from build123d import *

# Parameters (mm, degrees)
F1_DEPTH = 10
F2_DEPTH = 25
F3_R     = 7
F4_DEPTH = 60
F5_R     = 5


with BuildPart() as f1:
    # F0 (on Top) → F1 (new body)
    with BuildSketch(Plane.XY):
        Polygon((-115.381198, -8), (-4.618802, -8), (-9.237604, 0), (-4.618802, 8), (-115.381198, 8), align=None)
    extrude(amount=-F1_DEPTH)

    # F0 (on Top) → F2 (join)
    with BuildSketch(Plane.XY):
        Polygon((4.618802, -8), (9.237604, 0), (4.618802, 8), (-4.618802, 8), (-9.237604, 0), (-4.618802, -8), align=None)
        Polygon((2.453739, 4.25), (4.907477, 0), (2.453739, -4.25), (-2.453739, -4.25), (-4.907477, 0), (-2.453739, 4.25), align=None, mode=Mode.SUBTRACT)
    extrude(amount=-F2_DEPTH)

    # F3 (on face) → F4 (join)
    with BuildSketch(Plane(origin=(0, 0, -10), x_dir=(1, 0, 0), z_dir=(0, 0, -1))):
        with Locations((-107.381198, 0)):
            Circle(F3_R)
    extrude(amount=-F4_DEPTH)

    # F5
    f5_edges = [f1.edges().sort_by_distance(p)[0] for p in [
        (-114.381198, 0, 50),
    ]]
    fillet(f5_edges, radius=F5_R)


solid = f1.part
Work out the finished part from the listing and answer in its coordinate system (mm). A direction names the side the tool comes from. Give positions to 0.01 mm unless a question says otherwise; leave off trailing zeros. Loops run counter-clockwise (first coordinate to the right, second up) from the corner with the lowest first, then second, coordinate; pieces in that order, holes last. Notation, with made-up numbers: (-5.5, 58) -> (30.5, 58) arc R32 ccw to (30.5, 93) -> close; hole circle Ø5 at (73, 48.25). An arc over 180 degrees is marked (long way). Use a Markdown table: item, result. Add a question column.
1. Find the intervals of material crossed by probe 1 along Z at (x, y) = (-3, -5.5); probe 2 along Z at (x, y) = (-81, 7); probe 3 along X at (y, z) = (-0.5, -11), in increasing order.
2. For faces 4 (the flat face through (-6.896, 4.056, -17.395)), 5 (the flat face through (-6.961, -3.944, -17.395)), 6 (the cylindrical face through (-114.374, -0.308, 22.185)), 7 (the flat face through (-3.698, 2.095, -12.325)), 8 (the flat face through (-55, 8, -7)), determine the directions among +Z, -Z, +X, -X, +Y, -Y from which every point of the face is accessible in a straight line to the end or side of a thin tool.
3. Determine the mould class of faces 1 (the flat face through (-3.663, -2.155, -12.325)), 2 (the flat face through (4, 2, -25)), 3 (the flat face through (-115.381, 0, -5)) for opening direction X: released by +X, released by -X, zero draft, split by the parting line, or undercut.
4. Flat-ended cylindrical pins translate along their axes: pin 1 Ø6 at (y, z) = (0.5, 5) entering from -X; pin 2 Ø8 at (y, z) = (-6, 31) entering from +X; pin 3 Ø4 at (x, y) = (-53, 5) entering from -Z; pin 4 Ø6 at (x, y) = (-9, 4) entering from -Z. Find the tip coordinate at first contact, or state that the pin passes through.
5. Section A-A on x = -86.5 is taken. Determine the outline of the cut face in (y, z), and give its area (3 significant figures).
Results below:
| question | item | result |
|---|---|---|
| 1 | probe 1 | z = -25 to 0 |
| 1 | probe 2 | z = -10 to 0 |
| 1 | probe 3 | x = -8.95 to -4.62, 4.62 to 8.95 |
| 2 | face 4 | -Z, -X, +Y |
| 2 | face 5 | -Z, -X, -Y |
| 2 | face 6 | +Z |
| 2 | face 7 | +Z, -Z |
| 2 | face 8 | +Z, -Z, +X, -X, +Y |
| 3 | face 1 | undercut |
| 3 | face 2 | zero draft |
| 3 | face 3 | released by -X |
| 4 | pin 1 | stops at x = -114.38 |
| 4 | pin 2 | stops at x = -100.67 |
| 4 | pin 3 | stops at z = -10 |
| 4 | pin 4 | stops at z = -25 |
| 5 | outline | (-8, -10) -> (8, -10) -> (8, 0) -> (-8, 0) -> close |
| 5 | area | 160 mm^2 |
